Check sheet for the modelled part. Datum: model origin and axes. Units: mm. Face numbers are marked on the shaded views. A direction names the side the tool comes from. Coordinates: 2 decimals unless noted, no trailing zeros. Order: outer loops, then holes, each group sorted by start corner. A loop starts at its lowest first (then second) coordinate and runs counter-clockwise, first axis right, second up.
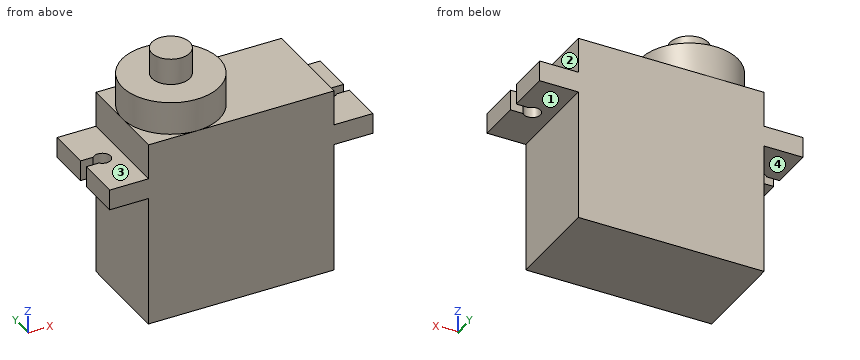
Autodesk Fusion 360 part; units mm, degrees
sketch "Sketch1" plane through (0, 0, 0) normal (0, 0, 1) x (1, 0, 0)
  line L0 (11.25, 5.9) -> (-11.25, 5.9)
  line L1 (-11.25, 5.9) -> (-11.25, -5.9)
  line L2 (-11.25, -5.9) -> (11.25, -5.9)
  line L3 (11.25, -5.9) -> (11.25, 5.9)
  line L4 (11.25, 5.9) -> (-11.25, -5.9) construction
  line L5 (-11.25, 5.9) -> (11.25, -5.9) construction
  dimension "d1" = 22.5
  dimension "d2" = 11.8
extrude "Extrude1" add sketch "Sketch1" along normal blind 22.7 makes body 1
sketch "Sketch2" plane through (0, 0, 0) normal (0, 0, 1) x (1, 0, 0)
sketch "Sketch3" plane through (0, 0, 0) normal (0, 0, 1) x (1, 0, 0)
  line L0 (-15.95, -5.9) -> (15.95, -5.9)
  line L1 (15.95, -5.9) -> (15.95, 5.9)
  line L2 (15.95, 5.9) -> (-15.95, 5.9)
  line L3 (-15.95, 5.9) -> (-15.95, -5.9)
  line L4 (-15.95, -5.9) -> (15.95, 5.9) construction
  line L5 (15.95, -5.9) -> (-15.95, 5.9) construction
  line L6 (-15.95, 0) -> (-15.95, -0.65) construction
  line L7 (-15.95, -0.65) -> (-13.65, -0.65)
  circle A0 centre (-13.65, 0) radius 1
  line L8 (-15.95, 0) -> (-15.95, 0.65) construction
  line L9 (-15.95, 0.65) -> (-13.65, 0.65)
  line L10 (15.95, 0) -> (15.95, -0.65) construction
  line L11 (15.95, -0.65) -> (13.65, -0.65)
  line L12 (15.95, 0) -> (15.95, 0.65)
  line L13 (15.95, 0.65) -> (13.65, 0.65)
  line L14 (13.65, -0.65) -> (13.65, 0.65) construction
  circle A1 centre (13.65, 0) radius 1
  line L15 (15.95, 0.65) -> (15.95, -0.65)
  line L16 (-15.95, 0.65) -> (-15.95, -0.65)
  dimension "d5" = 31.9
  dimension "d6" = 11.8
  dimension "d9" = 0.65
  dimension "d10" = 2.3
  dimension "d11" = 2
  dimension "d12" = 0.65
  dimension "d13" = 0.65
  dimension "d14" = 2.3
  dimension "d15" = 0.65
  dimension "d16" = 2.3
  dimension "d17" = 2
extrude "Extrude2" add sketch "Sketch3" along normal blind 2.5 separate body contours L0 L1 L2 L3 L7 A0 L9 L11 L13 A1 makes body 2
move_body "Move1" bodies 2 to x (1, 0, 0) y (0, 1, 0) z (0, 0, 1) at (0, 0, 15.9)
sketch "Sketch4" plane through (0, 0, 22.7) normal (0, 0, 1) x (-1, 0, 0)
  line L0 (-11.25, 5.9) -> (-11.25, -5.9)
  line L1 (-11.25, -5.9) -> (11.25, -5.9)
  line L2 (11.25, -5.9) -> (11.25, 5.9)
  line L3 (11.25, 5.9) -> (-11.25, 5.9)
  line L4 (11.25, 0) -> (5.35, 0) construction
  circle A0 centre (5.35, 0) radius 5.9
  dimension "d18" = 5.9
  dimension "d19" = 11.8
extrude "Extrude3" add sketch "Sketch4" along normal blind 4 contours A0 bodies 1
combine "Combine1" operation add target body 1 tool bodies 2
sketch "Sketch6" plane through (0, 0, 26.7) normal (0, 0, 1) x (-1, 0, 0)
  circle A0 centre (5.35, 0) radius 5.9
  circle A1 centre (5.35, 0) radius 2.3
  dimension "d22" = 4.6
extrude "Extrude4" add sketch "Sketch6" along normal blind 3.2 contours A1 bodies 1
(1) Cross-section at D-D (x = 3). Enter the section's corners in (y, z), and give its area (3 significant figures).
Filled in:
outline: (-5.9, 0) - (5.9, 0) - (5.9, 22.7) - (-5.9, 22.7) - close
area: 268 mm2
(2) Thickness scan on probe 1 along Y at (x, z) = (-13.65, 17.3); probe 2 along Z at (x, y) = (-1, 2); probe 3 along Z at (x, y) = (-12.5, 1.25). Record the ranges inside material, lowest first.
Filled in:
probe 1: y = -5.9 to -1, 1 to 5.9
probe 2: z = 0 to 26.7
probe 3: z = 15.9 to 18.4
(3) Cross-section at B-B (y = 1.75). Enter the section's corners in (x, z).
Filled in:
outline: (-15.95, 15.9) - (-11.25, 15.9) - (-11.25, 0) - (11.25, 0) - (11.25, 15.9) - (15.95, 15.9) - (15.95, 18.4) - (11.25, 18.4) - (11.25, 22.7) - (0.28, 22.7) - (0.28, 26.7) - (-3.86, 26.7) - (-3.86, 29.9) - (-6.84, 29.9) - (-6.84, 26.7) - (-10.98, 26.7) - (-10.98, 22.7) - (-11.25, 22.7) - (-11.25, 18.4) - (-15.95, 18.4) - close
(4) Cross-section at C-C (z = 23.25). Enter the section's corners in (x, y), and give its area (3 significant figures).
Filled in:
outline: circle Ø11.8 at (-5.35, 0)
area: 109 mm2
(5) Cross-section at A-A (x = -13.65). Enter the section's corners in (y, z).
Filled in:
outline: (-5.9, 15.9) - (-1, 15.9) - (-1, 18.4) - (-5.9, 18.4) - close; (1, 15.9) - (5.9, 15.9) - (5.9, 18.4) - (1, 18.4) - close
(6) Tool access check on the marked faces 1, 2, 3 and 4. Record the directions out of +Z, -Z, +X, -X, +Y, -Y that give a thin tool (end or side, any length) a straight path to the whole face; none if there is none.
Filled in:
face 1: -Z, +X, +Y, -Y
face 2: +Z, +X, +Y, -Y
face 3: +Z, -X, +Y, -Y
face 4: -Z, -X, +Y, -Y
(7) Go/stop test with flat-tipped pins: P1, Ø4.5, axis at y = 3, z = 21, coming from the -X side; P2, Ø3.5, axis at y = 0, z = 6.5, coming from the +X side; P3, Ø2, axis at x = 5, y = -1.5, coming from the +Z side. Record where each tip stops, or that it passes through.
Filled in:
P1: stops at x = -11.25
P2: stops at x = 11.25
P3: stops at z = 22.7
